```python
from build123d import *

# Parameters (mm, degrees)
F0_W     = 30
F0_H     = 30
F1_DEPTH = 1
F2_W     = 2.018653
F2_H     = 2.018654
F2_W_2   = 2.016375
F2_H_2   = 2.0191
F2_W_3   = 2.019964
F2_H_3   = 2.024288
F2_W_4   = 2.01923
F2_H_4   = 2.01923
F3_DEPTH = 0.5
F4_R     = 0.7


with BuildPart() as f1:
    # F0 (on Top) → F1 (new body)
    with BuildSketch(Plane.XY):
        with Locations((-26.442633, 11.425064)):
            Rectangle(F0_W, F0_H)
    extrude(amount=-F1_DEPTH)

    # F2 (on face) → F3 (join)
    with BuildSketch(Plane.XY):
        Polygon((-38.507011, 16.492767), (-38.507011, 6.388553), (-31.423131, -0.68813), (-21.315051, -0.68813), (-14.263901, 6.391955), (-14.263901, 16.494762), (-21.377073, 23.582622), (-31.424855, 23.582622), align=None)
        Polygon((-31.650189, 6.157815), (-31.650189, 0.719746), (-37.080094, 6.157815), align=None, mode=Mode.SUBTRACT)
        Polygon((-26.979655, 4.573753), (-30.809168, 0.727911), (-30.809168, 6.157815), (-28.563717, 6.157815), align=None, mode=Mode.SUBTRACT)
        Polygon((-33.854812, 11.440743), (-37.667993, 7.603067), (-37.667993, 15.286584), align=None, mode=Mode.SUBTRACT)
        Polygon((-31.666521, 6.998837), (-37.063763, 6.998837), (-33.23425, 10.836514), (-31.666521, 9.236122), align=None, mode=Mode.SUBTRACT)
        with Locations((-29.803097, 7.989094)):
            Rectangle(F2_W, F2_H, mode=Mode.SUBTRACT)
        Polygon((-26.981462, 8.58155), (-27.976304, 7.578057), (-27.976304, 9.014091), (-27.383724, 9.014091), align=None, mode=Mode.SUBTRACT)
        Polygon((-31.231981, 10.016147), (-32.637738, 11.439203), (-31.219007, 12.849177), (-29.809005, 11.421824), align=None, mode=Mode.SUBTRACT)
        Polygon((-28.805431, 9.843131), (-30.215511, 9.843131), (-29.212018, 10.829322), (-28.805431, 10.42706), align=None, mode=Mode.SUBTRACT)
        Polygon((-22.537747, 0.140012), (-30.213101, 0.140012), (-26.375424, 3.969523), align=None, mode=Mode.SUBTRACT)
        Polygon((-25.779359, 4.565588), (-24.195297, 6.157815), (-21.933518, 6.157815), (-21.933518, 0.703416), align=None, mode=Mode.SUBTRACT)
        Polygon((-15.695253, 6.157815), (-21.100661, 0.719746), (-21.100661, 6.157815), align=None, mode=Mode.SUBTRACT)
        Polygon((-27.769718, 6.581786), (-26.372593, 7.991966), (-24.962511, 6.56891), (-26.372533, 5.171744), align=None, mode=Mode.SUBTRACT)
        Polygon((-25.787652, 8.58155), (-25.368089, 9.001114), (-24.792811, 9.001114), (-24.792811, 7.586708), align=None, mode=Mode.SUBTRACT)
        with Locations((-22.940554, 7.998101)):
            Rectangle(F2_W_2, F2_H_2, mode=Mode.SUBTRACT)
        Polygon((-27.037146, 9.849087), (-27.982378, 10.779787), (-27.972091, 12.091455), (-27.011622, 13.036678), (-25.707053, 13.036678), (-24.78699, 12.102881), (-24.78699, 10.77085), (-25.736685, 9.849087), align=None, mode=Mode.SUBTRACT)
        Polygon((-23.960013, 9.843515), (-23.960013, 10.44087), (-23.527445, 10.845972), (-22.545587, 9.843515), align=None, mode=Mode.SUBTRACT)
        Polygon((-21.515666, 10.028902), (-22.936957, 11.45706), (-21.519115, 12.833655), (-20.115038, 11.422795), align=None, mode=Mode.SUBTRACT)
        Polygon((-21.108827, 7.015169), (-21.108827, 9.236122), (-19.516598, 10.84468), (-15.670758, 7.015169), align=None, mode=Mode.SUBTRACT)
        Polygon((-18.920535, 11.440744), (-15.074693, 15.294751), (-15.074693, 7.570407), align=None, mode=Mode.SUBTRACT)
        Polygon((-33.242416, 12.028642), (-37.055597, 15.874484), (-31.642023, 15.874484), (-31.642023, 13.620869), align=None, mode=Mode.SUBTRACT)
        Polygon((-29.207693, 12.036108), (-30.206861, 13.0223), (-28.818408, 13.0223), (-28.818408, 12.42972), align=None, mode=Mode.SUBTRACT)
        with Locations((-29.805265, 14.856238)):
            Rectangle(F2_W_3, F2_H_3, mode=Mode.SUBTRACT)
        Polygon((-27.381008, 13.859744), (-27.973332, 13.859744), (-27.977619, 15.258362), (-26.97318, 14.277282), align=None, mode=Mode.SUBTRACT)
        Polygon((-31.641971, 16.700408), (-37.086085, 16.700408), (-31.641971, 22.150441), align=None, mode=Mode.SUBTRACT)
        Polygon((-30.818034, 16.727873), (-30.818034, 22.145262), (-26.986726, 18.313954), (-28.579671, 16.727873), align=None, mode=Mode.SUBTRACT)
        Polygon((-23.534311, 12.02695), (-23.953147, 12.438918), (-23.953147, 13.036272), (-22.545587, 13.036272), align=None, mode=Mode.SUBTRACT)
        Polygon((-24.777411, 13.859262), (-25.37415, 13.859262), (-25.782874, 14.281611), (-24.777411, 15.281624), align=None, mode=Mode.SUBTRACT)
        Polygon((-26.382677, 14.877413), (-27.800711, 16.303259), (-26.380666, 17.707815), (-24.966487, 16.285844), align=None, mode=Mode.SUBTRACT)
        with Locations((-22.941211, 14.857687)):
            Rectangle(F2_W_4, F2_H_4, mode=Mode.SUBTRACT)
        Polygon((-19.523224, 12.038295), (-21.109303, 13.624375), (-21.109303, 15.862739), (-15.719378, 15.862739), align=None, mode=Mode.SUBTRACT)
        Polygon((-25.778282, 18.293355), (-21.933241, 22.152128), (-21.933241, 16.700408), (-24.185337, 16.700408), align=None, mode=Mode.SUBTRACT)
        Polygon((-26.375638, 18.890709), (-30.213814, 22.763215), (-22.551196, 22.763215), align=None, mode=Mode.SUBTRACT)
        Polygon((-21.109303, 16.714141), (-21.109303, 22.145262), (-15.678182, 16.714141), align=None, mode=Mode.SUBTRACT)
    extrude(amount=F3_DEPTH)

    # F4
    f4_edges = [f1.edges().sort_by_distance(p)[0] for p in [
        (-14.263901, 16.494762, 0.25),
        (-14.263901, 6.391955, 0.25),
        (-21.315051, -0.68813, 0.25),
        (-31.423131, -0.68813, 0.25),
        (-38.507011, 6.388553, 0.25),
        (-21.377073, 23.582622, 0.25),
        (-31.424855, 23.582622, 0.25),
        (-38.507011, 16.492767, 0.25),
    ]]
    fillet(f4_edges, radius=F4_R)


solid = f1.part
```
Can you work these out from the model? Positions are in its coordinate system, mm. A direction names the side the tool comes from. Coordinates: 2 decimals unless noted, no trailing zeros. Order: outer loops, then holes, each group sorted by start corner. A loop starts at its lowest first (then second) coordinate and runs counter-clockwise, first axis right, second up.
1. If we section it at D-D (x = -34.25): Please give me the cut outline in (y, z), then the cut area to 3 significant figures.
2. If we section it at C-C (y = -1.25): Please give me the cut outline in (x, z), then the cut area to 3 significant figures.
3. If we section it at A-A (x = -39.25): Please give me the cut outline in (y, z).
4. I need wall thicknesses on line 1 (X direction, y = 1, z = 0.05); line 2 (X direction, y = 17.5, z = 0.25); line 3 (Y direction, x = -16.5, z = 0.2). Which ranges of each line are inside material? Lowest first, please.
5. For faces 3 (the face through (-26.7, -3.575, -0.5)), 4 (the face through (-25.665, 15.591, 0.246)), which set-ups out of +Z, -Z, +X, -X, +Y, -Y let a thin tool reach every point of the face, with its end or its side?
6. I'm going to push a flat-ended pin straight in: pin 1 (1.6 mm diameter, centred on x = -27, y = 11, fed in from +Z). Where does the tip first touch, or does it pass through?
7. If we section it at B-B (y = 2): Please give me the cut outline in (x, z).
8. Thinking about a two-plate mould opening in Y: for faces 1 (the face through (-17.835, 2.806, 0.246)), 2 (the face through (-26, 16, 0)), which applies, +Y half, -Y half, draft (parallel to the pull), parting line (faces both ways), or undercut?
Entries:
1. outline: (-3.57, -1) - (26.43, -1) - (26.43, 0) - (20.75, 0) - (20.75, 0.5) - (19.54, 0.5) - (19.54, 0) - (16.7, 0) - (16.7, 0.5) - (15.87, 0.5) - (15.87, 0) - (13.04, 0) - (13.04, 0.5) - (11.84, 0.5) - (11.84, 0) - (11.04, 0) - (11.04, 0.5) - (9.82, 0.5) - (9.82, 0) - (7, 0) - (7, 0.5) - (6.16, 0.5) - (6.16, 0) - (3.32, 0) - (3.32, 0.5) - (2.14, 0.5) - (2.14, 0) - (-3.57, 0) - close
1. area: 33.2 mm2
2. outline: (-41.44, -1) - (-11.44, -1) - (-11.44, 0) - (-41.44, 0) - close
2. area: 30.0 mm2
3. outline: (-3.57, -1) - (26.43, -1) - (26.43, 0) - (-3.57, 0) - close
4. line 1: x = -33.11 to -31.93, -31.65 to -30.81, -30.54 to -29.35, -23.4 to -22.23, -21.93 to -21.1, -20.82 to -19.63
4. line 2: x = -37.5 to -36.29, -31.64 to -30.82, -27.8 to -26.59, -26.17 to -24.98, -21.93 to -21.11, -16.46 to -15.27
4. line 3: y = 4.15 to 5.35, 6.16 to 7.02, 7.84 to 9, 13.87 to 15.08, 15.86 to 16.71, 17.54 to 18.72
5. face 3: +Z, -Z, +X, -X, -Y
5. face 4: +Z
6. pin 1: stops at z = 0
7. outline: (-41.44, -1) - (-11.44, -1) - (-11.44, 0) - (-18.64, 0) - (-18.64, 0.5) - (-19.83, 0.5) - (-19.83, 0) - (-21.1, 0) - (-21.1, 0.5) - (-21.93, 0.5) - (-21.93, 0) - (-23.22, 0) - (-23.22, 0.5) - (-24.4, 0.5) - (-24.4, 0) - (-28.35, 0) - (-28.35, 0.5) - (-29.54, 0.5) - (-29.54, 0) - (-30.81, 0) - (-30.81, 0.5) - (-31.65, 0.5) - (-31.65, 0) - (-32.93, 0) - (-32.93, 0.5) - (-34.11, 0.5) - (-34.11, 0) - (-41.44, 0) - close
8. face 1: -Y half
8. face 2: undercut
